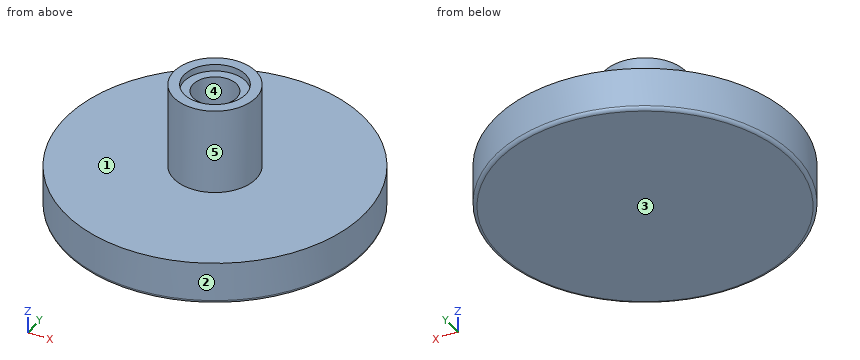
```python
from build123d import *

# Parameters (mm, degrees)
F0_R     = 11.1125
F0_R_2   = 3.048
F1_DEPTH = 3.175
F3_R     = 3.048
F4_DEPTH = 9.5504
F2_R     = 1.6129
F5_DEPTH = 25.4
F6_R     = 1.6129
F7_DEPTH = 3.175
F9_DEPTH = 0.508
F10_R    = 0.254


with BuildPart() as f1:
    # F0 (on Top) → F1 (new body)
    with BuildSketch(Plane.XY):
        Circle(F0_R)
        Circle(F0_R_2, mode=Mode.SUBTRACT)
    extrude(amount=F1_DEPTH)

    # F3 (on face) → F4 (join)
    with BuildSketch(Plane(origin=(0, 0, 0), x_dir=(1, 0, 0), z_dir=(0, 0, -1))):
        Circle(F3_R)
    extrude(amount=-F4_DEPTH)

    # F2 (on Top) → F5 (cut)
    with BuildSketch(Plane.XY):
        Circle(F2_R)
    extrude(amount=F5_DEPTH, mode=Mode.SUBTRACT)

    # F6 (on face) → F7 (join)
    with BuildSketch(Plane(origin=(0, 0, 0), x_dir=(1, 0, 0), z_dir=(0, 0, -1))):
        Circle(F6_R)
    extrude(amount=-F7_DEPTH)

    # F8 (on face) → F9 (cut)
    with BuildSketch(Plane.XY.offset(9.5504)):
        with BuildLine():
            ThreePointArc((2.286, 0), (0, 2.286), (-2.286, 0))
            ThreePointArc((-2.286, 0), (0, -2.286), (2.286, 0))
        make_face()
    extrude(amount=-F9_DEPTH, mode=Mode.SUBTRACT)

    # F10
    f10_edges = [f1.edges().sort_by_distance(p)[0] for p in [
        (-11.1125, 0, 0),
    ]]
    fillet(f10_edges, radius=F10_R)


solid = f1.part
```
Work out the finished part from the listing and answer in its coordinate system (mm). Face numbers are marked on the shaded views. A direction names the side the tool comes from. Give positions to 0.01 mm unless a question says otherwise; leave off trailing zeros. Loops run counter-clockwise (first coordinate to the right, second up) from the corner with the lowest first, then second, coordinate; pieces in that order, holes last. Notation, with made-up numbers: (82.5, 8.5) -> (115.5, 8.5) arc R18 cw to (115.5, 42.5) -> close; hole circle Ø10 at (88.25, -35). An arc over 180 degrees is marked (long way). Write item = value, one per line. Start each with the question number.
(1) Find section C-C on z = 2. Give the vertices of the cut face in (x, y) (1 decimal).
(2) The mould has two halves that part along X. Classify the marked faces 3, 4 and 5: +X half, -X half, draft (parallel to the pull), parting line (faces both ways), or undercut.
(3) Find the intervals of material crossed by probe 1 along Y at (x, z) = (0, 7.7); probe 2 along X at (y, z) = (0, 9.35), in increasing order. Write a range as from..to.
(4) Which of the six approach directions +Z, -Z, +X, -X, +Y, -Y give full straight-line access (tool end or side, diameter ignored) to the marked faces 1 and 2?
(5) Find section D-D on z = 6. Give the vertices of the cut face in (x, y).
(6) Given pin 1 Ø1.4 at (x, y) = (-0.5, -1) entering from +Z; pin 2 Ø3 at (x, y) = (-4, 7) entering from +Z (3 decimals), each flat-ended and moving along its own axis, determine where each tip first touches the part or whether it passes through.
From the geometry:
q1.outline = circle Ø22.2 at (0, 0)
q2.face_3 = draft
q2.face_4 = undercut
q2.face_5 = parting line
q3.probe_1 = -3.05..-1.61, 1.61..3.05
q3.probe_2 = -3.05..-2.29, 2.29..3.05
q4.face_1 = +Z
q4.face_2 = +Z, -Z
q5.outline = circle Ø6.1 at (0, 0); hole circle Ø3.23 at (0, 0)
q6.pin_1 = 9.04
q6.pin_2 = 3.175
